Check sheet for the modelled part. Datum: model origin and axes. Units: mm. A direction names the side the tool comes from. Give positions to 0.01 mm unless a question says otherwise; leave off trailing zeros. Write each loop counter-clockwise with the first axis right and the second up, starting at its lowest first coordinate (ties: lowest second). Pieces come first, ordered by that corner, then holes. Notation, with made-up numbers: (26, 1.5) -> (82, 1.5) arc R14 ccw to (82, 13.5) -> close; hole circle Ø2 at (85.25, 46). An arc over 180 degrees is marked (long way). Return JSON: item names as keys, results as strings.
from build123d import *

# Parameters (mm, degrees)
F0_W     = 25.4
F0_H     = 25.4
F1_DEPTH = 292.1
F2_R     = 3.175
F3_T     = 3.175


# Not quite as in the source:
# - a shell that OpenCascade refuses in one call is made with other operations: the cavity is built on its own and cut out


with BuildPart() as f1:
    # F0 (on Front) → F1 (new body)
    with BuildSketch(Plane.XZ):
        Rectangle(F0_W, F0_H)
    extrude(amount=F1_DEPTH)

    # F2
    f2_edges = [f1.edges().sort_by_distance(p)[0] for p in [
        (-12.7, -146.05, 12.7),
        (12.7, -146.05, 12.7),
        (12.7, -146.05, -12.7),
        (-12.7, -146.05, -12.7),
    ]]
    fillet(f2_edges, radius=F2_R)

    # F3: shell of thickness 3.175, made by hand


with BuildPart() as f3_core1:
    # F3_t2: copy of F1
    add(f1.part)

    # the walls: a layer under each face that stays
    f3_faces = [f3_core1.faces().sort_by_distance(p)[0] for p in [
        (0, -146.05, -12.7),
        (-12.7, -146.05, 0),
        (12.7, -146.05, 0),
        (0, -146.05, 12.7),
    ]]
    thicken(f3_faces, amount=-F3_T, mode=Mode.SUBTRACT)


with BuildPart() as f1_1:
    add(f1.part)

    # what is left inside the walls is the cavity
    f3_cavity = [f3_core1.part.solids().sort_by_distance(p)[0] for p in [
        (0, -194.733333, -9.49325),
    ]]
    add(f3_cavity, mode=Mode.SUBTRACT)


solid = f1_1.part
(1) Set-up check for faces 4 (the flat face through (11, -292.1, 0)), 5 (the flat face through (0, -144, 9.525)): record each of +Z, -Z, +X, -X, +Y, -Y from which the full face is reachable in a straight line by a thin tool's end or side.
Reply:
{"face 4": "+Z, -Z, +X, -X, -Y", "face 5": "+Y, -Y"}
(2) Cross-section at B-B on y = -36. Enter the section's corners in (x, z) (3 decimals), then the cut area to 3 significant figures.
Reply:
{"outline": "(-12.7, -9.525) arc R3.175 ccw to (-9.525, -12.7) -> (9.525, -12.7) arc R3.175 ccw to (12.7, -9.525) -> (12.7, 9.525) arc R3.175 ccw to (9.525, 12.7) -> (-9.525, 12.7) arc R3.175 ccw to (-12.7, 9.525) -> close; hole (-9.525, -9.525) -> (9.525, -9.525) -> (9.525, 9.525) -> (-9.525, 9.525) -> close", "area": "274 mm^2"}
(3) Release check for a two-part mould opening along X. For faces 1 (the flat face through (-12.7, -144, 0)), 2 (the flat face through (11, 0, 0)), 3 (the flat face through (9.525, -144, 0)) record: pulls with the +X half, pulls with the -X half, needs draft (parallel to the pull), parting line crosses it, or undercut.
Reply:
{"face 1": "pulls with the -X half", "face 2": "needs draft", "face 3": "undercut"}
(4) Cross-section at C-C on z = -2.5. Enter the section's corners in (x, y) (3 decimals), then the cut area to 3 significant figures.
Reply:
{"outline": "(-12.7, -292.1) -> (-9.525, -292.1) -> (-9.525, 0) -> (-12.7, 0) -> close; (9.525, -292.1) -> (12.7, -292.1) -> (12.7, 0) -> (9.525, 0) -> close", "area": "1,850 mm^2"}
(5) Thickness scan on L1, parallel to Z at x = 8.25, y = -20 (3 decimals); L2, parallel to Z at x = -10.25, y = -29. Record the ranges inside material, lowest first.
Reply:
{"L1": "-12.7 to -9.525, 9.525 to 12.7", "L2": "-12.62 to 12.62"}
(6) Cross-section at A-A on x = 5. Enter the section's corners in (y, z) (3 decimals).
Reply:
{"outline": "(-292.1, -12.7) -> (0, -12.7) -> (0, -9.525) -> (-292.1, -9.525) -> close; (-292.1, 9.525) -> (0, 9.525) -> (0, 12.7) -> (-292.1, 12.7) -> close"}
